Print and shaded views of the part. All mm, measured from the part's lowest x, y and z. Round coordinates to 2 decimals unless told otherwise and drop trailing zeros. Order: outer loops, then holes, each group sorted by start corner. A loop starts at its lowest first (then second) coordinate and runs counter-clockwise, first axis right, second up. Notation, with made-up numbers: (76, -34.75) - (133, -34.75) arc R21 ccw to (133, -20.75) - close; hole circle Ø9 at (0, -26.75). An arc over 180 degrees is marked (long way). Return JSON: item names as keys, results as strings. Group by question number.
Item 1: Probe probe 1 along X at (y, z) = (5, 2.2); probe 2 along Y at (x, z) = (4.95, 2.9); probe 3 along Y at (x, z) = (4.25, 2.65). List the from-to ranges inside material, lowest first.
Item 2: Saw through at A-A on y = 5. List the corners of the cut face in (x, z), and give its area (3 significant figures).
Item 3: Saw through at C-C on z = 2.5. List the corners of the cut face in (x, y).
Item 4: Drop a flat-ended pin along its axis: pin 1 (3 mm diameter, centred on x = 4.95, y = 5, fed in from -Z). Give the stop position or say it passes through.
Item 5: Saw through at B-B on x = 4.95. List the corners of the cut face in (y, z).
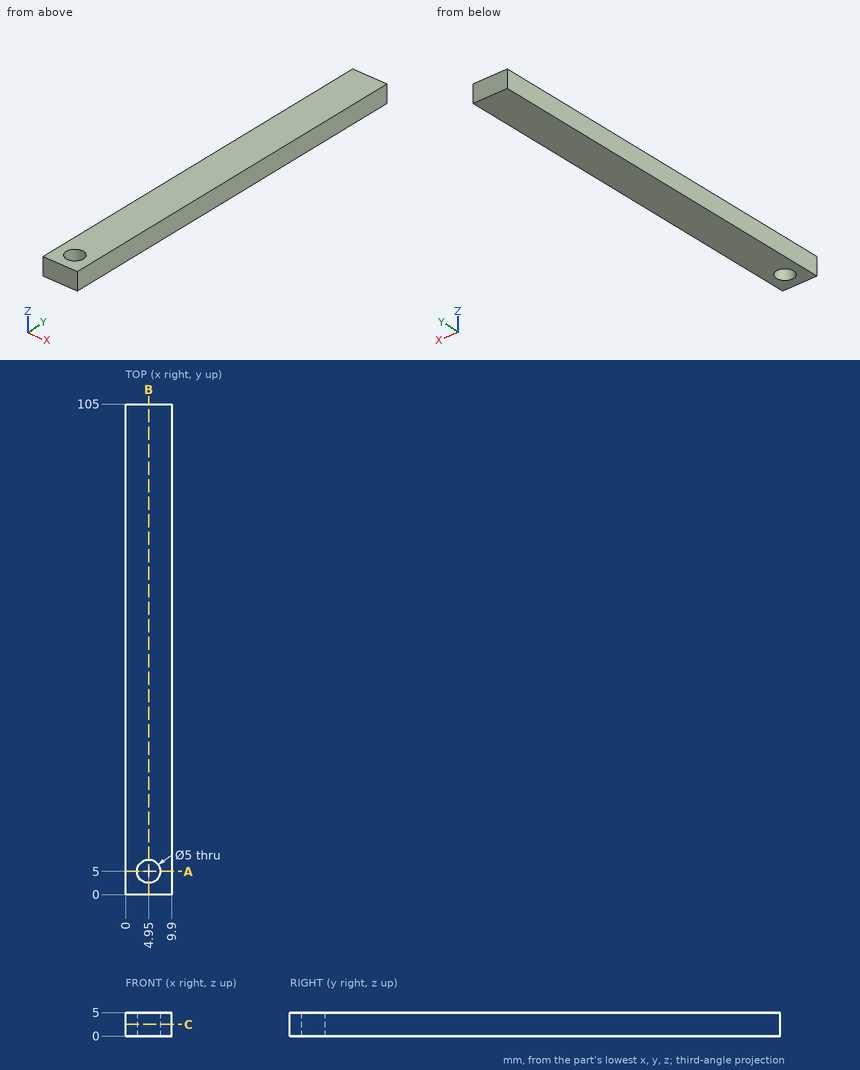
Filled in:
{
 "1": {"probe 1": "x = 0 to 2.45, 7.45 to 9.9", "probe 2": "y = 0 to 2.5, 7.5 to 105", "probe 3": "y = 0 to 2.6, 7.4 to 105"},
 "2": {"outline": "(0, 0) - (2.45, 0) - (2.45, 5) - (0, 5) - close; (7.45, 0) - (9.9, 0) - (9.9, 5) - (7.45, 5) - close", "area": "24.5 mm^2"},
 "3": {"outline": "(0, 0) - (9.9, 0) - (9.9, 105) - (0, 105) - close; hole circle Ø5 at (4.95, 5)"},
 "4": {"pin 1": "passes through"},
 "5": {"outline": "(0, 0) - (2.5, 0) - (2.5, 5) - (0, 5) - close; (7.5, 0) - (105, 0) - (105, 5) - (7.5, 5) - close"}
}
